from build123d import *

# Parameters (mm, degrees)
SKETCH_1_W      = 20
SKETCH_1_H      = 20
SKETCH_1_R      = 1
EXTRUDE_1_DEPTH = 3


with BuildPart() as part:
    # 草图1 → 凸台-拉伸1 (new body)
    with BuildSketch(Plane.XY):
        Rectangle(SKETCH_1_W, SKETCH_1_H)
        with Locations((4, 4.75)):
            Circle(SKETCH_1_R, mode=Mode.SUBTRACT)
        with Locations((4, -4.75)):
            Circle(SKETCH_1_R, mode=Mode.SUBTRACT)
        with BuildLine():
            Line((-6, 5.75), (-2, 5.75))
            ThreePointArc((-2, 5.75), (-1, 4.75), (-2, 3.75))
            Line((-2, 3.75), (-6, 3.75))
            ThreePointArc((-6, 3.75), (-7, 4.75), (-6, 5.75))
        make_face(mode=Mode.SUBTRACT)
        with BuildLine():
            Line((-6, -5.75), (-2, -5.75))
            ThreePointArc((-2, -5.75), (-1, -4.75), (-2, -3.75))
            Line((-2, -3.75), (-6, -3.75))
            ThreePointArc((-6, -3.75), (-7, -4.75), (-6, -5.75))
        make_face(mode=Mode.SUBTRACT)
    extrude(amount=EXTRUDE_1_DEPTH)


solid = part.part
Source: CAD feature listing. Evaluate the final solid. Frame: model axes, mm. A direction names the side the tool comes from. Coordinates: 2 decimals unless noted, no trailing zeros. Loops run counter-clockwise (first coordinate to the right, second up) from the corner with the lowest first, then second, coordinate; pieces in that order, holes last. Notation, with made-up numbers: (-12, -4.5) -> (37, -4.5) arc R33 ccw to (37, 29.5) -> close; hole circle Ø11 at (15, 59). An arc over 180 degrees is marked (long way). Answer in a Markdown table with one row per item. Add a question column.
Q1. Section A-A on x = -5.5. Return the cut outline in (y, z).
Q2. Reachability of faces 1 (the face through (0, 10, 1)), 2 (the face through (-7, 4.7, 1.5)) from +Z, -Z, +X, -X, +Y, -Y: full face, straight path, thin tool, end or side. Return the list, or none.
Q3. Section B-B on y = -4.75. Return the cut outline in (x, z).
Q4. Ray query, line 1 along Y through (x, z) = (-2, 0.7); line 2 along X through (y, z) = (5, 0.95). Return the intervals inside material, ascending.
Q5. Section C-C on z = 2.6. Return the cut outline in (x, y).
Q6. Pull-direction query (Y, two-part tool) for faces 3 (the face through (10, 0, 1)), 4 (the face through (0, -10, 1)), 5 (the face through (-4, 5.75, 1)); classes: pulls with the +Y half, pulls with the -Y half, needs draft (parallel to the pull), parting line crosses it, or undercut.
Computed values:
| question | item | result |
|---|---|---|
| 1 | outline | (-10, 0) -> (-5.75, 0) -> (-5.75, 3) -> (-10, 3) -> close; (-3.75, 0) -> (3.75, 0) -> (3.75, 3) -> (-3.75, 3) -> close; (5.75, 0) -> (10, 0) -> (10, 3) -> (5.75, 3) -> close |
| 2 | face 1 | +Z, -Z, +X, -X, +Y |
| 2 | face 2 | +Z, -Z |
| 3 | outline | (-10, 0) -> (-7, 0) -> (-7, 3) -> (-10, 3) -> close; (-1, 0) -> (3, 0) -> (3, 3) -> (-1, 3) -> close; (5, 0) -> (10, 0) -> (10, 3) -> (5, 3) -> close |
| 4 | line 1 | y = -10 to -5.75, -3.75 to 3.75, 5.75 to 10 |
| 4 | line 2 | x = -10 to -6.97, -1.03 to 3.03, 4.97 to 10 |
| 5 | outline | (-10, -10) -> (10, -10) -> (10, 10) -> (-10, 10) -> close; hole (-6, -5.75) -> (-2, -5.75) arc R1 ccw to (-2, -3.75) -> (-6, -3.75) arc R1 ccw to start; hole (-6, 3.75) -> (-2, 3.75) arc R1 ccw to (-2, 5.75) -> (-6, 5.75) arc R1 ccw to start; hole circle Ø2 at (4, -4.75); hole circle Ø2 at (4, 4.75) |
| 6 | face 3 | needs draft |
| 6 | face 4 | pulls with the -Y half |
| 6 | face 5 | undercut |
